```python
from build123d import *


with BuildPart() as part:
    # Sketch1 → Revolve1 (revolve)
    with BuildSketch(Plane.XY, mode=Mode.PRIVATE) as revolve1_sk:
        with BuildLine():
            Line((0, 316.674418605), (0, 314.174418605))
            Line((0, 314.174418605), (86, 314.174418605))
            Line((86, 314.174418605), (86, 276.174418605))
            Line((86, 276.174418605), (81, 276.174418605))
            Line((81, 276.174418605), (81, 309.174418605))
            Line((81, 309.174418605), (-5, 309.174418605))
            Line((-5, 309.174418605), (-5, 314.134629268))
            ThreePointArc((-5, 314.134629268), (-21.02740861, 313.469956125), (-37, 311.988085198))
            Line((-37, 311.988085198), (-37, 314.505464815))
            ThreePointArc((-37, 314.505464815), (-18.53175896, 316.131715126), (0, 316.674418605))
        make_face()
    revolve(revolve1_sk.sketch.rotate(Axis((86, 276.174418605, 0), (-1, 0, 0)), 90), axis=Axis((86, 276.174418605, 0), (-1, 0, 0)))


solid = part.part
```
Here's how the part is built. I have some questions about the finished solid (model axes, mm). A direction names the side the tool comes from. Give positions to 0.01 mm unless a question says otherwise; leave off trailing zeros. Order: outer loops, then holes, each group sorted by start corner. A loop starts at its lowest first (then second) coordinate and runs counter-clockwise, first axis right, second up. Notation, with made-up numbers: (17, 7.25) -> (31, 7.25) arc R24 cw to (31, 41.25) -> close; hole circle Ø4 at (-3, 73.5). An arc over 180 degrees is marked (long way). Use CSV: the item, a comma, the result in double quotes. Start each with the question number.
Item 1: I'm going to push flat-ended pins straight in: P1, Ø23, axis at y = 264, z = -2.5, coming from the -X side; P2, Ø5, axis at x = 56.5, z = 16, coming from the +Y side; P3, Ø6, axis at x = 25.5, y = 255.5, coming from the +Z side. Where does each tip first touch, or does it pass through?
Item 2: Thinking about a two-plate mould opening in X: for faces 4 (the flat face through (86, 276, 1)), 5 (the flat face through (-5, 242, 0)), 6 (the flat face through (81, 276, 0)), which applies, pulls with the +X half, pulls with the -X half, needs draft (parallel to the pull), parting line crosses it, or undercut?
Item 3: If I drill on probe 1 along Y at (x, z) = (40, 0); probe 2 along X at (y, z) = (244.5, 15); probe 3 along X at (y, z) = (298, -12), over which ranges is the centre line in solid material (lowest first)? Write a range as [from, to].
Item 4: On a 3-axis mill with a long thin cutter (end or side, diameter ignored), from which of +Z, -Z, +X, -X, +Y, -Y can I reach the whole of each face in a straight line? I mean faces 1 (the flat face through (-37, 242, -12)), 2 (the cylindrical face through (37.398, 243.455, 4.296)), 3 (the cylindrical face through (43.6, 313.27, 8.24)). Say none if no direction works.
Item 5: Suppose I cut it at A-A (x = 74). List the corners of the cut face in (y, z) for me.
Answer block:
1,P1,"stops at x = 81"
1,P2,"stops at y = 311.7"
1,P3,"stops at z = 33.64"
2,face 4,"pulls with the +X half"
2,face 5,"undercut"
2,face 6,"pulls with the -X half"
3,probe 1,"y = [238.17, 243.17], [309.17, 314.17]"
3,probe 2,"x = [-5, 86]"
3,probe 3,"x = [81, 86]"
4,face 1,"+Z, -Z, -X, +Y, -Y"
4,face 2,"-X"
4,face 3,"+X"
5,outline,"circle Ø76 at (276.17, 0); hole circle Ø66 at (276.17, 0)"
